```python
from build123d import *

# Parameters (mm, degrees)
F0_R     = 32.5
F0_W     = 45
F0_H     = 26
F1_DEPTH = 1
F2_W     = 2.5
F2_H     = 12
F2_W_2   = 5
F2_H_2   = 2.5
F3_DEPTH = 3
F4_SIZE  = 2


with BuildPart() as f1:
    # F0 (on Top) → F1 (new body)
    with BuildSketch(Plane.XY):
        Circle(F0_R)
        Rectangle(F0_W, F0_H, mode=Mode.SUBTRACT)
    extrude(amount=F1_DEPTH)

    # F2 (on face) → F3 (join)
    with BuildSketch(Plane.XY.offset(1)):
        with Locations((0, 19)):
            Rectangle(F2_W, F2_H)
        with Locations((0, -19)):
            Rectangle(F2_W, F2_H)
        with Locations((-25, 0)):
            Rectangle(F2_W_2, F2_H_2)
        with Locations((25, 0)):
            Rectangle(F2_W_2, F2_H_2)
    extrude(amount=F3_DEPTH)

    # F4
    f4_edges = [f1.edges().sort_by_distance(p)[0] for p in [
        (-22.5, 0, 4),
        (22.5, 0, 4),
        (0, 13, 4),
        (0, -13, 4),
    ]]
    chamfer(f4_edges, length=F4_SIZE)


solid = f1.part
```
Part model, mm, in its own coordinate system. A direction names the side the tool comes from. Coordinates: 2 decimals unless noted, no trailing zeros. Write each loop counter-clockwise with the first axis right and the second up, starting at its lowest first coordinate (ties: lowest second). Pieces come first, ordered by that corner, then holes.
Item 1: Slice it at D-D (y = -7.5). Write the cut outline in (x, z).
Item 2: Mould opens along Y. For faces 1 (the face through (-22.5, 0, 1)), 2 (the face through (0, 13, 1)), 3 (the face through (0, 20, 4)), 4 (the face through (0, -25, 2)) say: released by +Y, released by -Y, zero draft, split by the parting line, or undercut.
Item 3: Probe line 1 (Y direction, x = -23.5, z = 2.8); line 2 (Y direction, x = -10, z = 0.85); line 3 (Y direction, x = 3, z = 0.5). List the from-to ranges inside material, lowest first.
Item 4: Slice it at A-A (x = 0). Write the cut outline in (y, z).
Item 5: Slice it at B-B (y = 0). Write the cut outline in (x, z).
Item 6: Which spindle directions (+Z, -Z, +X, -X, +Y, -Y) get a long thin tool onto all of the face, cutting with end or side? Do faces 5 (the face through (0, 14, 3)), 6 (the face through (23.5, 0, 3)), 7 (the face through (0, 25, 2)), 8 (the face through (1.25, -19, 2)), 9 (the face through (-1.25, 19, 2)). Say none if no direction does.
Item 7: Slice it at C-C (y = 14). Write the cut outline in (x, z), and give its area (3 significant figures).
Item 8: Pin check, flat tips, straight feed: pin 1 (1.5 mm diameter, centred on y = -17.5, z = 3, fed in from -X); pin 2 (2 mm diameter, centred on x = -0.5, z = 3, fed in from +Y); pin 3 (1.5 mm diameter, centred on x = -24, z = 3, fed in from -Y). Stop position of each tip, or through.
Results found:
1. outline: (-31.62, 0) - (-22.5, 0) - (-22.5, 1) - (-31.62, 1) - close; (22.5, 0) - (31.62, 0) - (31.62, 1) - (22.5, 1) - close
2. face 1: undercut
2. face 2: undercut
2. face 3: zero draft
2. face 4: released by -Y
3. line 1: y = -1.25 to 1.25
3. line 2: y = -30.92 to -13, 13 to 30.92
3. line 3: y = -32.36 to -13, 13 to 32.36
4. outline: (-32.5, 0) - (-13, 0) - (-13, 2) - (-15, 4) - (-25, 4) - (-25, 1) - (-32.5, 1) - close; (13, 0) - (32.5, 0) - (32.5, 1) - (25, 1) - (25, 4) - (15, 4) - (13, 2) - close
5. outline: (-32.5, 0) - (-22.5, 0) - (-22.5, 2) - (-24.5, 4) - (-27.5, 4) - (-27.5, 1) - (-32.5, 1) - close; (22.5, 0) - (32.5, 0) - (32.5, 1) - (27.5, 1) - (27.5, 4) - (24.5, 4) - (22.5, 2) - close
6. face 5: +Z, +X, -X
6. face 6: +Z, +Y, -Y
6. face 7: +Z, +X, -X, +Y
6. face 8: +Z, +X, +Y, -Y
6. face 9: +Z, -X, +Y, -Y
7. outline: (-29.33, 0) - (29.33, 0) - (29.33, 1) - (1.25, 1) - (1.25, 3) - (-1.25, 3) - (-1.25, 1) - (-29.33, 1) - close
7. area: 63.7 mm2
8. pin 1: stops at x = -1.25
8. pin 2: stops at y = 25
8. pin 3: stops at y = -1.25
